For this review, take the finished solid that the model builds, in its own axes (mm). Give positions to 0.01 mm unless a question says otherwise; leave off trailing zeros. Order: outer loops, then holes, each group sorted by start corner. A loop starts at its lowest first (then second) coordinate and runs counter-clockwise, first axis right, second up. Notation, with made-up numbers: (48.5, -23.75) - (78.5, -23.75) arc R23 ccw to (78.5, -9.75) - close; hole circle Ø2 at (76.5, 51). An arc over 180 degrees is marked (long way). Use a Markdown table: item, result. Add a question column.
1) Clearance check with flat-ended pins moving along their axes: P1, Ø1, axis at y = -16.5, z = -37.5, coming from the +X side; P2, Ø5, axis at y = -21.5, z = 74, coming from the +X side; P3, Ø1.5, axis at x = -54.5, y = -14.5, coming from the -Z side. State where each tip first meets the part, or that it passes through.
2) We need section B-B on y = -15.75. Write out the cut boundary in (x, z), then the cut area to 3 significant figures.
3) We need section C-C on z = -20. Write out the cut boundary in (x, y), then the cut area to 3 significant figures.
4) We need section A-A on x = 0. Write out the cut boundary in (y, z).
5) Wall thickness on L1, parallel to Z at x = -12.5, y = -1.25; L2, parallel to Z at x = -13, y = -7.25 (3 decimals); L3, parallel to X at y = -13.5, z = -10: over which ranges is each line inside the solid? List them lowest first.
6) Mouldability with a two-part tool opening along X and no side actions: class faces 1 (the face through (-28.59, -12.32, 107.13)), 2 (the face through (0, -12, -75)), 3 (the face through (24.192, -12.325, 17.944)) as released by +X, released by -X, zero draft, split by the parting line, or undercut.
7) We need section D-D on z = -43. Write out the cut boundary in (x, y).
```python
from build123d import *

# Parameters (mm, degrees)
F0_R     = 45
F1_DEPTH = 25
F2_R     = 50
F3_R     = 70
F4_R     = 20


with BuildPart() as f1:
    # F0 (on Front) → F1 (new body)
    with BuildSketch(Plane.XZ):
        with BuildLine():
            Line((0, 125), (-80, 75))
            Line((-80, 75), (-30.923292, 75))
            ThreePointArc((-30.923292, 75), (0, 97.5), (30.923292, 75))
            Line((30.923292, 75), (80, 75))
            Line((80, 75), (0, 125))
        make_face()
        with BuildLine():
            Line((-30.923292, 75), (-80, 75))
            Line((-80, 75), (-80, -75))
            Line((-80, -75), (80, -75))
            Line((80, -75), (80, 75))
            Line((80, 75), (30.923292, 75))
            ThreePointArc((30.923292, 75), (32.103403, 70.061769), (32.5, 65))
            ThreePointArc((32.5, 65), (-5.061769, 32.896597), (-30.923292, 75))
        make_face()
        with Locations((0, -20)):
            Circle(F0_R, mode=Mode.SUBTRACT)
    extrude(amount=F1_DEPTH)

    # F2
    f2_edges = [f1.edges().sort_by_distance(p)[0] for p in [
        (-80, -12.5, -75),
        (80, -12.5, -75),
    ]]
    fillet(f2_edges, radius=F2_R)

    # F3
    f3_edges = [f1.edges().sort_by_distance(p)[0] for p in [
        (80, -12.5, 75),
        (-80, -12.5, 75),
    ]]
    fillet(f3_edges, radius=F3_R)

    # F4
    f4_edges = [f1.edges().sort_by_distance(p)[0] for p in [
        (0, -12.5, 125),
    ]]
    fillet(f4_edges, radius=F4_R)


solid = f1.part
```
Checked values:
| question | item | result |
|---|---|---|
| 1 | P1 | x = 78.54 |
| 1 | P2 | x = 70.45 |
| 1 | P3 | z = -69 |
| 2 | outline | (-80, -25) arc R50 ccw to (-30, -75) - (30, -75) arc R50 ccw to (80, -25) - (80, 36.2) arc R70 ccw to (47.1, 95.56) - (10.6, 118.38) arc R20 ccw to (-10.6, 118.38) - (-47.1, 95.56) arc R70 ccw to (-80, 36.2) - close; hole circle Ø90 at (0, -20); hole (30.92, 75) arc R32.5 ccw (long way) to (32.5, 65) arc R32.5 ccw to start |
| 2 | area | 16,700 mm² |
| 3 | outline | (-80, -25) - (-45, -25) - (-45, 0) - (-80, 0) - close; (45, -25) - (80, -25) - (80, 0) - (45, 0) - close |
| 3 | area | 1,750 mm² |
| 4 | outline | (-25, -75) - (0, -75) - (0, -65) - (-25, -65) - close; (-25, 25) - (0, 25) - (0, 32.5) - (-25, 32.5) - close; (-25, 97.5) - (0, 97.5) - (0, 121.42) - (-25, 121.42) - close |
| 5 | L1 | -75 to -63.23, 23.23 to 35, 95 to 117.19 |
| 5 | L2 | -75 to -63.081, 23.081 to 35.213, 94.787 to 116.875 |
| 5 | L3 | -80 to -43.87, 43.87 to 80 |
| 6 | face 1 | released by -X |
| 6 | face 2 | zero draft |
| 6 | face 3 | undercut |
| 7 | outline | (-76.65, -25) - (-38.68, -25) - (-38.68, 0) - (-76.65, 0) - close; (38.68, -25) - (76.65, -25) - (76.65, 0) - (38.68, 0) - close |
